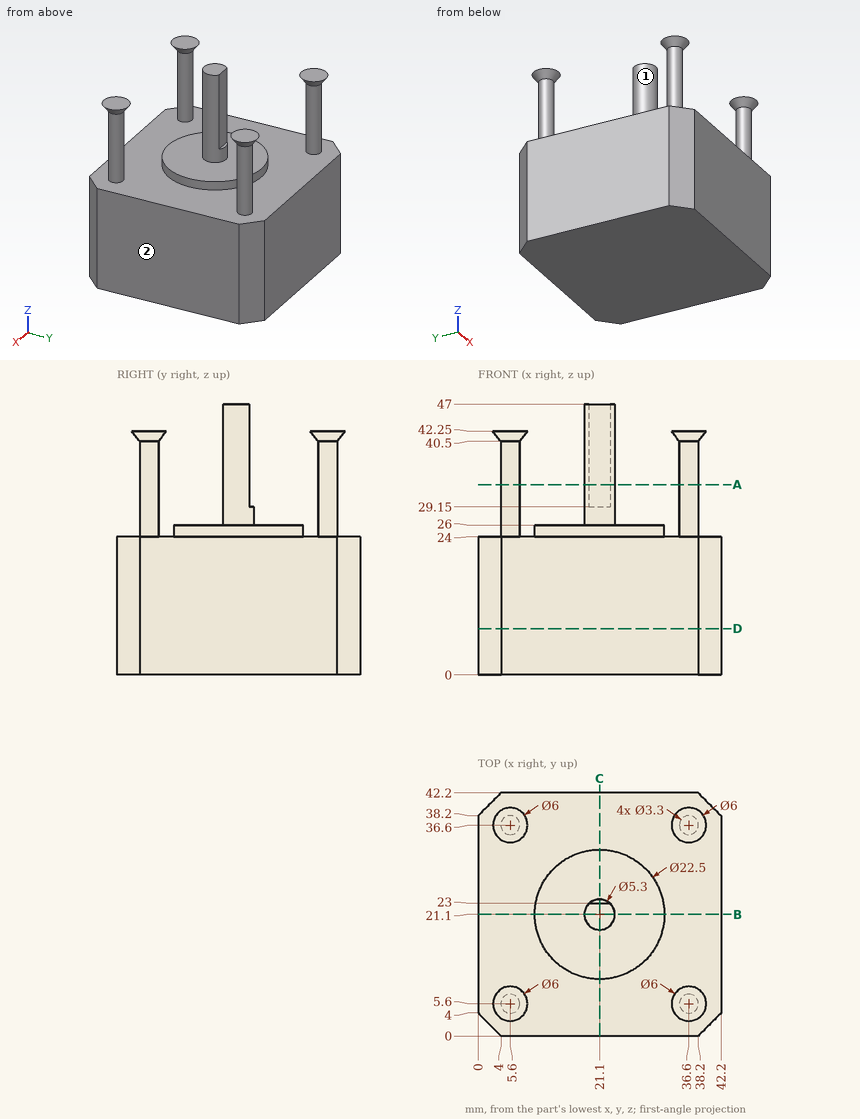
Answer from the drawing. Dimensions are ordinates in mm from the lowest x, y and z of the part. A direction names the side the tool comes from. Coordinates: 2 decimals unless noted, no trailing zeros. Write each loop counter-clockwise with the first axis right and the second up, starting at its lowest first coordinate (ties: lowest second). Pieces come first, ordered by that corner, then holes. Notation, with made-up numbers: M -3.75,69.5 L 33.25,69.5 A11 cw 33.25,74.5 Z; hole C -36.5,-6.5 d8. An arc over 180 degrees is marked long. Use one line per item in the form item = value. Start each with the question number.
1. The part is cut by section C-C (x = 21.1). Give the vertices of the cut face in (y, z).
2. A tool of negligible diameter and unlimited length cuts with its end or side. For the marked faces 1 and 2, from which of +Z, -Z, +X, -X, +Y, -Y can it reach the whole face along a straight path? Write none if from no direction.
3. Straight lines are drawn through the part: probe 1 along Z at (x, y) = (31, 3); probe 2 along Z at (x, y) = (38, 7.5); probe 3 along X at (y, z) = (38.5, 42). For each, find the intervals that lie inside material, in ascending order. Write a range as from..to.
4. The part is cut by section D-D (z = 8). Give the vertices of the cut face in (x, y), plus the area to 3 significant figures.
5. The part is cut by section A-A (z = 33). Give the vertices of the cut face in (x, y).
6. The part is cut by section B-B (y = 21.1). Give the vertices of the cut face in (x, z).
7. Each of these flat-tipped pins is pushed along its axis until it touches: P1, Ø4, axis at x = 22, z = 38.5, coming from the +Y side; P2, Ø5, axis at x = 37, y = 36.5, coming from the +Z side; P3, Ø10, axis at y = 10.5, z = 32, coming from the +X side. Where does it stop, or does it pass through?
Evaluation:
q1.outline = M 0,0 L 42.2,0 L 42.2,24 L 32.35,24 L 32.35,26 L 23.75,26 L 23.75,29.15 L 23,29.15 L 23,47 L 18.45,47 L 18.45,26 L 9.85,26 L 9.85,24 L 0,24 Z
q2.face_1 = +Z
q2.face_2 = +Z, -Z, +X, +Y, -Y
q3.probe_1 = 0..24
q3.probe_2 = 0..24, 41.42..42.25
q3.probe_3 = 3.53..7.67, 34.53..38.67
q4.outline = M 0,4 L 4,0 L 38.2,0 L 42.2,4 L 42.2,38.2 L 38.2,42.2 L 4,42.2 L 0,38.2 Z
q4.area = 1,750 mm^2
q5.outline = C 5.6,5.6 d3.3; C 5.6,36.6 d3.3; M 19.25,23 A2.65 ccw long 22.95,23 Z; C 36.6,5.6 d3.3; C 36.6,36.6 d3.3
q6.outline = M 0,0 L 42.2,0 L 42.2,24 L 32.35,24 L 32.35,26 L 23.75,26 L 23.75,47 L 18.45,47 L 18.45,26 L 9.85,26 L 9.85,24 L 0,24 Z
q7.P1 = 23
q7.P2 = 42.25
q7.P3 = 38.25
